Read the model definition and answer for the solid it produces. Units are mm, in the model's axes. Face numbers are marked on the shaded views. A direction names the side the tool comes from. Coordinates: 2 decimals unless noted, no trailing zeros. Loops run counter-clockwise (first coordinate to the right, second up) from the corner with the lowest first, then second, coordinate; pieces in that order, holes last. Notation, with made-up numbers: (-24, 43.5) - (31, 43.5) arc R10 cw to (31, 48.5) - close; hole circle Ø11 at (5.5, -31.75). An arc over 180 degrees is marked (long way). One line per question, with ' | ' between items. Start each with the question number.
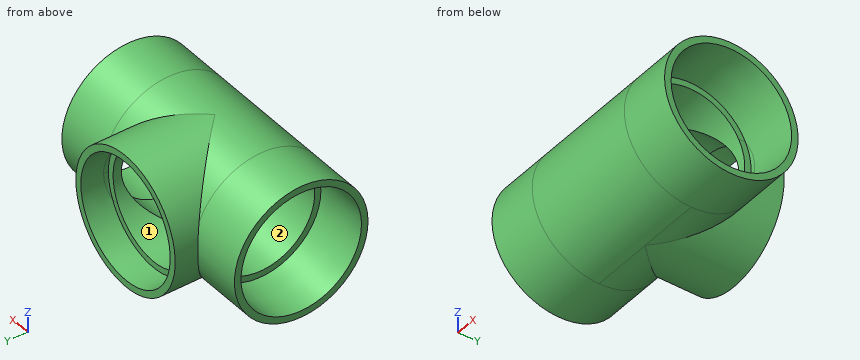
```python
from build123d import *

# Parameters (mm, degrees)
SKETCH4_R           = 63.6016
BOSS_EXTRUDE1_DEPTH = 117.9576
SKETCH5_R           = 63.6016
BOSS_EXTRUDE2_DEPTH = 58.9788
SKETCH8_R           = 92.190098926
SKETCH8_R_2         = 25.050168183
CUT_EXTRUDE1_DEPTH  = 25.4


with BuildPart() as part:
    # Sketch1 → Revolve1 (revolve)
    with BuildSketch(Plane.XY):
        Polygon((-110.5154, -63.6016), (-58.9788, -63.6016), (-58.9788, -57.0357), (-110.5154, -57.3786), align=None)
        Polygon((110.5154, -57.3786), (58.9788, -57.0357), (58.9788, -63.6016), (110.5154, -63.6016), align=None)
    revolve(axis=Axis((-110.5154, 0, 0), (1, 0, 0)))



with BuildPart() as body_2:
    # Sketch2 → Revolve2 (revolve)
    with BuildSketch(Plane.XY):
        Polygon((57.3786, 110.5154), (57.0357, 58.9788), (63.6016, 58.9788), (63.6016, 110.5154), align=None)
    revolve(axis=Axis((0, 0, 0), (0, 1, 0)))


with BuildPart() as part_1:
    add(part.part)

    add(body_2.part)  # Boss-Extrude1 merges body 2
    # Sketch4 → Boss-Extrude1 (add)
    with BuildSketch(Plane(origin=(-58.9788, 0, 0), x_dir=(0, 0, -1), z_dir=(1, 0, 0))):
        Circle(SKETCH4_R)
    extrude(amount=BOSS_EXTRUDE1_DEPTH)

    # Sketch5 → Boss-Extrude2 (add)
    with BuildSketch(Plane.XZ.offset(-58.9788)):
        Circle(SKETCH5_R)
    extrude(amount=BOSS_EXTRUDE2_DEPTH)

    # Sketch6 → Cut-Revolve1 (revolve, cut)
    with BuildSketch(Plane.XY):
        Polygon((-110.5154, -57.3786), (-58.9788, -57.0357), (-58.9788, -51.1302), (58.9788, -51.1302), (58.9788, -57.0357), (110.5154, -57.3786), (110.5154, 0), (-110.5154, 0), align=None)
    revolve(axis=Axis((110.5154, 0, 0), (-1, 0, 0)), mode=Mode.SUBTRACT)

    # Sketch7 → Cut-Revolve2 (revolve, cut)
    with BuildSketch(Plane.XY):
        Polygon((57.3786, 110.5154), (57.0357, 58.9788), (51.1302, 58.9788), (51.1302, 0), (0, 0), (0, 110.5154), align=None)
    revolve(axis=Axis((0, 0, 0), (0, 1, 0)), mode=Mode.SUBTRACT)

    # Sketch8 → Cut-Extrude1 (cut)
    with BuildSketch(Plane(origin=(0, 110.5154, 0), x_dir=(1, 0, 0), z_dir=(0, 1, 0))):
        Circle(SKETCH8_R)
        Circle(SKETCH8_R_2, mode=Mode.SUBTRACT)
    extrude(amount=-CUT_EXTRUDE1_DEPTH, mode=Mode.SUBTRACT)


solid = part_1.part
```
1) The part is cut by section C-C on y = 72.5. Write down the section's boundary in (x, z), and give its area (3 significant figures).
2) Find the intervals of material crossed by line 1 along Z through (x, y) = (0, 15); line 2 along Y through (x, z) = (-25, 0); line 3 along Z through (x, y) = (-97, 12.5), in increasing order. Write a range as from..to.
3) The part is cut by section B-B on x = 82.5. Write down the section's boundary in (y, z).
4) Which of the six approach directions +Z, -Z, +X, -X, +Y, -Y give full straight-line access (tool end or side, diameter ignored) to the marked faces 1 and 2?
5) Given pin 1 Ø6 at (y, z) = (49.5, -0.5) entering from +X; pin 2 Ø1.5 at (x, y) = (-72, -32.5) entering from -Z; pin 3 Ø3 at (x, z) = (50, 19) entering from -Y, each flat-ended and moving along its own axis, determine where each tip first touches the part or whether it passes through.
6) The part is cut by section A-A on z = -40. Count the separate pieces of the cut face and the enclosed holes in it, and give its area (3 significant figures).
Answer below:
1) outline: circle Ø127.2 at (0, 0); hole circle Ø114.25 at (0, 0) | area: 2,460 mm2
2) line 1: -63.6..-51.13, 51.13..63.6 | line 2: -63.6..-51.13 | line 3: -62.36..-55.91, 55.91..62.36
3) outline: circle Ø127.2 at (0, 0); hole circle Ø114.38 at (0, 0)
4) face 1: +Y | face 2: +X, -X
5) pin 1: x = 58.98 | pin 2: z = -55.11 | pin 3: y = -61.15
6) separate pieces: 3 | enclosed holes: 0 | area: 5,580 mm2
